Check sheet for the drawn part. Datum: minimum x, y, z corner. Units: mm. Round coordinates to 2 decimals unless told otherwise and drop trailing zeros. Order: outer loops, then holes, each group sorted by start corner. A loop starts at its lowest first (then second) coordinate and runs counter-clockwise, first axis right, second up. Notation, with made-up numbers: M -11,-23 L 43,-23 A19 ccw 43,-6 Z; hole C -8,39.5 d6. An arc over 180 degrees is marked long. Use one line per item in the form item = value. Start each with the question number.
Item 1: Cross-section at C-C on y = 3. Enter the section's corners in (x, z) (1 decimal).
Item 2: Thickness scan on probe 1 along Y at (x, z) = (2.9, 5.5); probe 2 along X at (y, z) = (2.4, 2) (1 decimal); probe 3 along Y at (x, z) = (1.85, 3) (1 decimal). Record the ranges inside material, lowest first. Write a range as [from, to].
Item 3: Cross-section at D-D on x = 5.35. Enter the section's corners in (y, z), then the cut area to 3 significant figures.
Item 4: Go/stop test with flat-tipped pins: pin 1 Ø1.5 at (y, z) = (0.5, 3.5) entering from -X; pin 2 Ø1.5 at (x, z) = (5, 1.5) entering from -Y; pin 3 Ø1 at (y, z) = (1.5, 4.5) entering from +X (1 decimal). Record where each tip stops, or that it passes through.
Item 5: Cross-section at A-A on z = 2. Enter the section's corners in (x, y), then the cut area to 3 significant figures.
Item 6: Release check for a two-part mould opening along X. For the marked faces 1, 2, 3 and 4 record: +X half, -X half, draft (parallel to the pull), parting line (faces both ways), or undercut.
Item 7: Cross-section at B-B on x = 3.75. Enter the section's corners in (y, z).
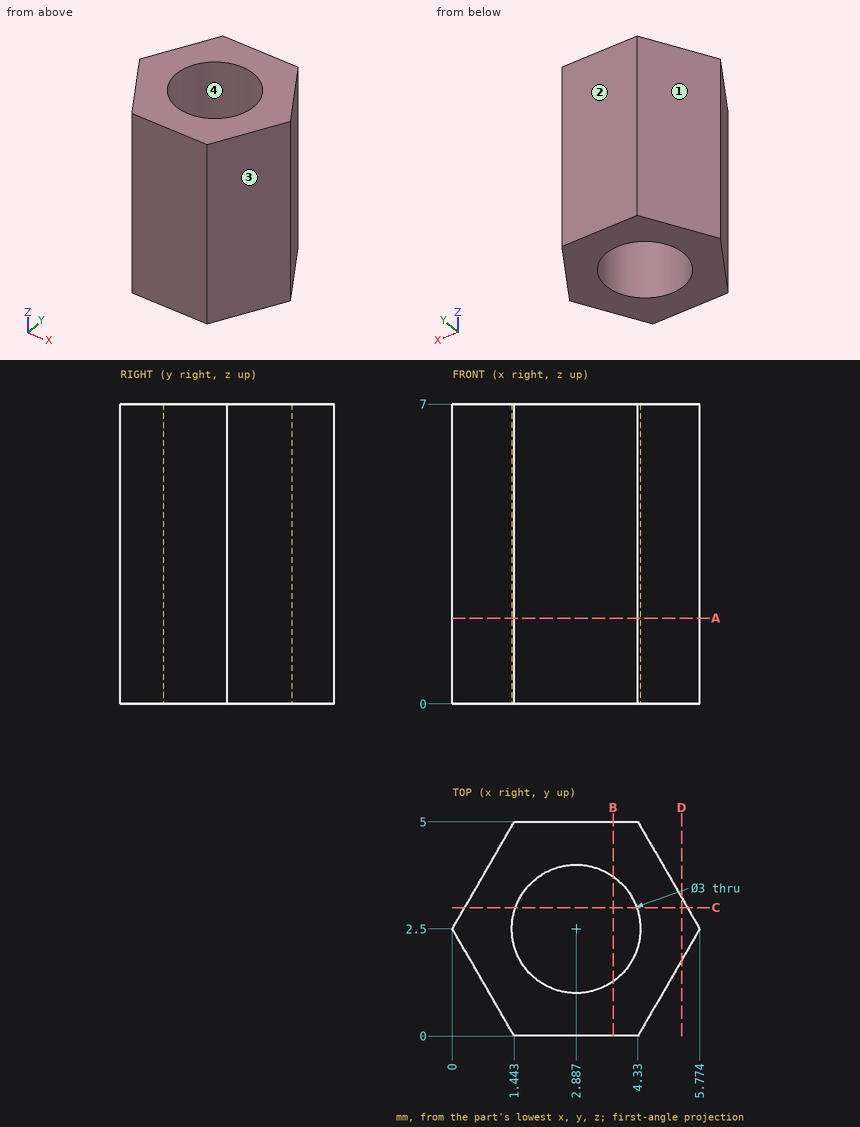
Output values:
q1.outline = M 0.3,0 L 1.5,0 L 1.5,7 L 0.3,7 Z; M 4.3,0 L 5.5,0 L 5.5,7 L 4.3,7 Z
q2.probe_1 = [0, 1], [4, 5]
q2.probe_2 = [0.1, 1.4], [4.4, 5.7]
q2.probe_3 = [0, 1.4], [3.6, 5]
q3.outline = M 1.77,0 L 3.23,0 L 3.23,7 L 1.77,7 Z
q3.area = 10.3 mm2
q4.pin_1 = 0.72
q4.pin_2 = 0
q4.pin_3 = 5.5
q5.outline = M 0,2.5 L 1.44,0 L 4.33,0 L 5.77,2.5 L 4.33,5 L 1.44,5 Z; hole C 2.89,2.5 d3
q5.area = 14.6 mm2
q6.face_1 = -X half
q6.face_2 = draft
q6.face_3 = +X half
q6.face_4 = undercut
q7.outline = M 0,0 L 1.27,0 L 1.27,7 L 0,7 Z; M 3.73,0 L 5,0 L 5,7 L 3.73,7 Z
